Part model, mm, in its own coordinate system. Round coordinates to 2 decimals unless told otherwise and drop trailing zeros. Write each loop counter-clockwise with the first axis right and the second up, starting at its lowest first coordinate (ties: lowest second). Pieces come first, ordered by that corner, then holes.
1) Saw through at A-A on z = 304.8. Write the cut outline in (x, y), and give its area (3 significant figures).
2) Saw through at C-C on y = 30.5. Write the cut outline in (x, z), and give its area (3 significant figures).
3) Saw through at B-B on x = 20. Write the cut outline in (y, z), and give its area (3 significant figures).
4) Saw through at D-D on z = 78. Write the cut outline in (x, y).
5) Drill centre lines: L1, parallel to Y at x = 33.5, z = 76; L2, parallel to X at y = 22, z = 180; L3, parallel to X at y = 46, z = 304. Where is each one in solid material? Low to high.
6) Flat gauge pins, fed straight in: pin 1 (10 mm diameter, centred on x = 16, y = 43, fed in from +Z); pin 2 (4 mm diameter, centred on x = 55, y = 22, fed in from -Z); pin 3 (11.5 mm diameter, centred on x = 37.04, z = 304.8, fed in from -Y); pin 4 (1.5 mm diameter, centred on x = 41.5, y = 5.5, fed in from -Z). Where does each tip first touch, or does it go through?
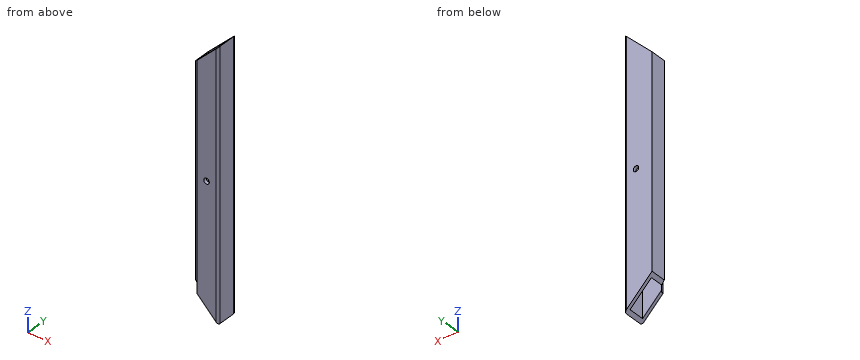
```python
from build123d import *

# Parameters (mm, degrees)
F0_W      = 63.5
F0_H      = 50.8
F1_DEPTH  = 609.6
F3_DEPTH  = 76.2
F5_R      = 15.0324721588
F6_DEPTH  = 609.6
F7_R      = 5.08
F8_R      = 6.35
F9_DEPTH  = 76.2
F4_W      = 49.2759997249
F4_H      = 36.5759997249
F10_DEPTH = 609.6


with BuildPart() as f1:
    # F0 (on Top) → F1 (new body)
    with BuildSketch(Plane.XY):
        with Locations((31.75, 25.4)):
            Rectangle(F0_W, F0_H)
    extrude(amount=F1_DEPTH)

    # F2 (on face) → F3 (cut)
    with BuildSketch(Plane(origin=(0, 50.8, 0), x_dir=(-1, 0, 0), z_dir=(0, 1, 0))):
        Polygon((13.9825628959, 77.4825628959), (0, 63.5), (0, 0), (40.1009321213, 0), align=None)
        Polygon((0, 63.5), (-63.5, 0), (0, 0), align=None)
        Polygon((0, 609.6), (-63.5, 609.6), (0, 546.1), align=None)
    extrude(amount=-F3_DEPTH, mode=Mode.SUBTRACT)

    # F5 (on Top) → F6 (cut)
    with BuildSketch(Plane.XY):
        Circle(F5_R)
    extrude(amount=F6_DEPTH, mode=Mode.SUBTRACT)

    # F7
    f7_edges = [f1.edges().sort_by_distance(p)[0] for p in [
        (63.5, 50.8, 304.8),
        (63.5, 0, 304.8),
    ]]
    fillet(f7_edges, radius=F7_R)

    # F8 (on face) → F9 (cut)
    with BuildSketch(Plane.XZ):
        with Locations((37.0356701314, 304.8)):
            Circle(F8_R)
    extrude(amount=-F9_DEPTH, mode=Mode.SUBTRACT)

    # F4 (on Top) → F10 (cut)
    with BuildSketch(Plane.XY):
        with Locations((31.75, 25.4)):
            Rectangle(F4_W, F4_H)
    extrude(amount=F10_DEPTH, mode=Mode.SUBTRACT)


solid = f1.part
```
Completed:
1. outline: (0, 15.03) arc R15.03 cw to (7.11, 13.24) - (7.11, 43.69) - (30.69, 43.69) - (30.69, 50.8) - (0, 50.8) - close; (13.24, 7.11) arc R15.03 cw to (15.03, 0) - (30.69, 0) - (30.69, 7.11) - close; (43.39, 0) - (58.42, 0) arc R5.08 ccw to (63.5, 5.08) - (63.5, 45.72) arc R5.08 ccw to (58.42, 50.8) - (43.39, 50.8) - (43.39, 43.69) - (56.39, 43.69) - (56.39, 7.11) - (43.39, 7.11) - close
1. area: 1,080 mm2
2. outline: (0, 63.5) - (7.11, 56.39) - (7.11, 553.21) - (0, 546.1) - close; (56.39, 7.11) - (63.5, 0) - (63.5, 609.6) - (56.39, 602.49) - close
2. area: 7,770 mm2
3. outline: (0, 43.5) - (7.11, 43.5) - (7.11, 566.1) - (0, 566.1) - close; (43.69, 43.5) - (50.8, 43.5) - (50.8, 566.1) - (43.69, 566.1) - close
3. area: 7,430 mm2
4. outline: (0, 15.03) arc R15.03 cw to (7.11, 13.24) - (7.11, 43.69) - (56.39, 43.69) - (56.39, 7.11) - (13.24, 7.11) arc R15.03 cw to (15.03, 0) - (58.42, 0) arc R5.08 ccw to (63.5, 5.08) - (63.5, 45.72) arc R5.08 ccw to (58.42, 50.8) - (0, 50.8) - close
5. L1: y = 0 to 7.11, 43.69 to 50.8
5. L2: x = 0 to 7.11, 56.39 to 63.5
5. L3: x = 0 to 30.74, 43.34 to 63.49
6. pin 1: stops at z = 567.05
6. pin 2: stops at z = 6.5
6. pin 3: passes through
6. pin 4: stops at z = 21.25
